The model under review builds one solid part; all positions refer to its coordinate system, in mm. Face numbers are marked on the shaded views. A direction names the side the tool comes from. Coordinates: 2 decimals unless noted, no trailing zeros. Write each loop counter-clockwise with the first axis right and the second up, starting at its lowest first coordinate (ties: lowest second). Pieces come first, ordered by that corner, then holes. Notation, with made-up numbers: (0, -32.75) - (7, -32.75) arc R29 ccw to (7, -8.75) - close; hole circle Ø9 at (-21, 87). An arc over 180 degrees is marked (long way). Put each result on its own line as item: value. Start each with the question number.
Item 1: For pin 1 (6.5 mm diameter, centred on y = 47, z = 7.5, fed in from -X); pin 2 (2.5 mm diameter, centred on x = -11.875, z = 7.5, fed in from +Y); pin 3 (3 mm diameter, centred on x = -20.5, z = 6.5, fed in from -Y), all flat-tipped, find the tip position at first contact; note any pin that passes through.
Item 2: Consider section D-D on y = 36.5. Give the boundary of the cut face in (x, z).
Item 3: To check wall thickness, follow L1, parallel to X at y = 44.75, z = 7.5 (3 decimals); L2, parallel to X at y = 30, z = 1.5; L3, parallel to X at y = -31, z = 13 (3 decimals). State the ranges of each line that lie inside material, in increasing order. Write a range as [from, to].
Item 4: Consider section C-C on y = -27.5. Give the boundary of the cut face in (x, z).
Item 5: Machinability: for the marked faces 4, 5, 6 and 7, which of the approach directions +Z, -Z, +X, -X, +Y, -Y give a long, thin tool a straight path to every point of the face, cutting with its end or side? Answer none if there is none.
Item 6: Mouldability with a two-part tool opening along X and no side actions: class the marked faces 1, 2 and 3 as pulls with the +X half, pulls with the -X half, needs draft (parallel to the pull), parting line crosses it, or undercut.
Item 7: Consider section A-A on z = 7.5. Give the boundary of the cut face in (x, y) (3 decimals), then the cut area to 3 significant figures.
Item 8: Consider section B-B on z = 1.75. Give the boundary of the cut face in (x, y), then the cut area to 3 significant figures.
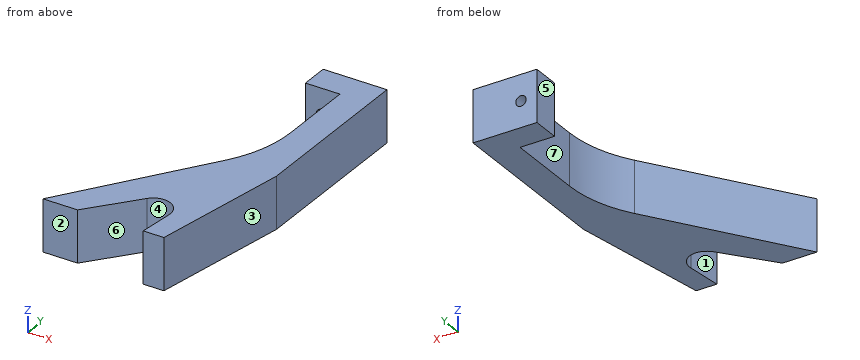
```python
from build123d import *

# Parameters (mm, degrees)
BOSS_EXTRUDE1_DEPTH = 15
SKETCH2_R           = 1.5
CUT_EXTRUDE1_DEPTH  = 15


with BuildPart() as part:
    # Sketch1 → Boss-Extrude1 (new body)
    with BuildSketch(Plane.XY):
        with BuildLine():
            Line((-11, 42), (-6.5, 42))
            Line((-6.5, 42), (-6.5, 19.663584609))
            ThreePointArc((-6.5, 19.663584609), (-8.071080696, 9.29500929), (-12.643277381, -0.1427164))
            Line((-12.643277381, -0.1427164), (-40, -40))
            Line((-40, -40), (-30, -40))
            Line((-30, -40), (-18.772519607, -26.233092947))
            ThreePointArc((-18.772519607, -26.233092947), (-12.972906424, -24.778489823), (-9.925888036, -29.923104703))
            Line((-9.925888036, -29.923104703), (-11, -40))
            Line((-11, -40), (-5, -40))
            Line((-5, -40), (2, 0))
            Line((2, 0), (2, 30))
            Line((2, 30), (2, 50))
            Line((2, 50), (-11, 50))
            Line((-11, 50), (-16.5, 50))
            Line((-16.5, 50), (-16.5, 42))
            Line((-16.5, 42), (-11, 42))
        make_face()
    extrude(amount=BOSS_EXTRUDE1_DEPTH)

    # Sketch2 → Cut-Extrude1 (cut)
    with BuildSketch(Plane(origin=(0, 50, 0), x_dir=(1, 0, 0), z_dir=(0, 1, 0))):
        with Locations(Location((-11.875, -7.5, 0), (0, 0, 270))):
            Circle(SKETCH2_R)
    extrude(amount=-CUT_EXTRUDE1_DEPTH, mode=Mode.SUBTRACT)


solid = part.part
```
Report:
1. pin 1: x = -16.5
1. pin 2: y = 3.18
1. pin 3: y = -30.19
2. outline: (-6.5, 0) - (2, 0) - (2, 15) - (-6.5, 15) - close
3. L1: [-16.5, -13.375], [-10.375, 2]
3. L2: [-6.5, 2]
3. L3: [-33.823, -22.66], [-10.041, -3.425]
4. outline: (-31.42, 0) - (-19.81, 0) - (-19.81, 15) - (-31.42, 15) - close; (-10.27, 0) - (-2.81, 0) - (-2.81, 15) - (-10.27, 15) - close
5. face 4: +Z, -Z
5. face 5: +Z, -Z, -X, +Y
5. face 6: +Z, -Z, -Y
5. face 7: +Z, -Z, -X
6. face 1: undercut
6. face 2: needs draft
6. face 3: pulls with the +X half
7. outline: (-40, -40) - (-30, -40) - (-18.773, -26.233) arc R5 cw to (-9.926, -29.923) - (-11, -40) - (-5, -40) - (2, 0) - (2, 50) - (-10.375, 50) - (-10.375, 42) - (-6.5, 42) - (-6.5, 19.664) arc R35 cw to (-12.643, -0.143) - close; (-16.5, 42) - (-13.375, 42) - (-13.375, 50) - (-16.5, 50) - close
7. area: 1,310 mm²
8. outline: (-40, -40) - (-30, -40) - (-18.77, -26.23) arc R5 cw to (-9.93, -29.92) - (-11, -40) - (-5, -40) - (2, 0) - (2, 50) - (-16.5, 50) - (-16.5, 42) - (-6.5, 42) - (-6.5, 19.66) arc R35 cw to (-12.64, -0.14) - close
8. area: 1,330 mm²
